from build123d import *

# Parameters (mm, degrees)
SKETCH1_W               = 5
SKETCH1_H               = 13
SKETCH1_R               = 1.25
BOSS_EXTRUDE1_DEPTH     = 2.5
BOSS_EXTRUDE1_2_DEPTH   = 2.5
SKETCH1_5_W             = 32.5
SKETCH1_5_H             = 2
BOSS_EXTRUDE2_DEPTH     = 20.5
SKETCH1_6_W             = 32.5
SKETCH1_6_H             = 3
BOSS_EXTRUDE3_DEPTH     = 3.5
SKETCH2_R               = 1.5
CUT_EXTRUDE2_DEPTH      = 14
CUT_EXTRUDE2_DEPTH_BACK = 8


with BuildPart() as part:
    # Sketch1 → Boss-Extrude1 (new body)
    with BuildSketch(Plane.XY):
        with Locations((-13.75, 6.5)):
            Rectangle(SKETCH1_W, SKETCH1_H)
        with Locations((-13.75, 6)):
            Circle(SKETCH1_R, mode=Mode.SUBTRACT)
    extrude(amount=BOSS_EXTRUDE1_DEPTH)



with BuildPart() as body_2:
    # Sketch1 → Boss-Extrude1 2 (new body)
    with BuildSketch(Plane.XY):
        with Locations((13.75, 6.5)):
            Rectangle(SKETCH1_W, SKETCH1_H)
        with Locations((13.75, 6)):
            Circle(SKETCH1_R, mode=Mode.SUBTRACT)
    extrude(amount=BOSS_EXTRUDE1_2_DEPTH)


with BuildPart() as part_1:
    add(part.part)

    add(body_2.part)  # Boss-Extrude2 merges body 2
    # Sketch1<5> → Boss-Extrude2 (add)
    with BuildSketch(Plane.XY):
        with Locations((0, -1)):
            Rectangle(SKETCH1_5_W, SKETCH1_5_H)
        with Locations((0, -6)):
            Rectangle(SKETCH1_5_W, SKETCH1_5_H)
    extrude(amount=BOSS_EXTRUDE2_DEPTH)

    # Sketch1<6> → Boss-Extrude3 (add)
    with BuildSketch(Plane.XY):
        with Locations((0, -3.5)):
            Rectangle(SKETCH1_6_W, SKETCH1_6_H)
    extrude(amount=BOSS_EXTRUDE3_DEPTH)

    # Sketch2 → Cut-Extrude2 (cut, two sides)
    with BuildSketch(Plane(origin=(0, 0, 0), x_dir=(1, 0, 0), z_dir=(0, 1, 0))) as cut_extrude2_sk:
        with Locations((13.75, -8.5)):
            Circle(SKETCH2_R)
        with Locations((13.75, -15.5)):
            Circle(SKETCH2_R)
        with Locations((-13.75, -15.5)):
            Circle(SKETCH2_R)
        with Locations((-13.75, -8.5)):
            Circle(SKETCH2_R)
    extrude(amount=CUT_EXTRUDE2_DEPTH, mode=Mode.SUBTRACT)
    extrude(cut_extrude2_sk.sketch, amount=-CUT_EXTRUDE2_DEPTH_BACK, mode=Mode.SUBTRACT)


solid = part_1.part
Geometry: final body of the model. Coordinates: model frame, mm. A direction names the side the tool comes from. Coordinates: 2 decimals unless noted, no trailing zeros. Write each loop counter-clockwise with the first axis right and the second up, starting at its lowest first coordinate (ties: lowest second). Pieces come first, ordered by that corner, then holes. Notation, with made-up numbers: (2.5, 5) - (53.5, 5) arc R19 ccw to (53.5, 22) - close; hole circle Ø10 at (-13.5, 74.5). An arc over 180 degrees is marked (long way). Return JSON: item names as keys, results as strings.
Item 1: Line query: L1, parallel to X at y = -0.95, z = 8.5; L2, parallel to Z at x = -13.75, y = -1.2; L3, parallel to Y at x = 10, z = 17.25. Output: solid intervals per line, ascending.
Completed:
{"L1": "x = -16.25 to -15.25, -12.25 to 12.25, 15.25 to 16.25", "L2": "z = 0 to 7, 10 to 14, 17 to 20.5", "L3": "y = -7 to -5, -2 to 0"}
Item 2: Section query A-A (z = 19). Output: boundary loops of the cut face in (x, y), and give its area (3 significant figures).
Completed:
{"outline": "(-16.25, -7) - (16.25, -7) - (16.25, -5) - (-16.25, -5) - close; (-16.25, -2) - (16.25, -2) - (16.25, 0) - (-16.25, 0) - close", "area": "130 mm2"}
Item 3: Section query B-B (y = 2.75). Output: boundary loops of the cut face in (x, z), and give its area (3 significant figures).
Completed:
{"outline": "(-16.25, 0) - (-11.25, 0) - (-11.25, 2.5) - (-16.25, 2.5) - close; (11.25, 0) - (16.25, 0) - (16.25, 2.5) - (11.25, 2.5) - close", "area": "25.0 mm2"}
Item 4: Pull-direction query (X, two-part tool) for faces 1 (the face through (-14, 13, 1)), 2 (the face through (16.25, -1, 8)), 3 (the face through (12.56, -0.99, 9.41)); classes: +X half, -X half, draft (parallel to the pull), parting line (faces both ways), or undercut.
Completed:
{"face 1": "draft", "face 2": "+X half", "face 3": "undercut"}
Item 5: Section query D-D (z = 15.5). Output: boundary loops of the cut face in (x, y).
Completed:
{"outline": "(-16.25, -7) - (-15.25, -7) - (-15.25, -5) - (-16.25, -5) - close; (-16.25, -2) - (-15.25, -2) - (-15.25, 0) - (-16.25, 0) - close; (-12.25, -7) - (12.25, -7) - (12.25, -5) - (-12.25, -5) - close; (-12.25, -2) - (12.25, -2) - (12.25, 0) - (-12.25, 0) - close; (15.25, -7) - (16.25, -7) - (16.25, -5) - (15.25, -5) - close; (15.25, -2) - (16.25, -2) - (16.25, 0) - (15.25, 0) - close"}
Item 6: Section query C-C (x = -13.75). Count the separate pieces of the cut face and the enclosed holes in it, and give its area (4 significant figures).
Completed:
{"separate pieces": "6", "enclosed holes": "0", "area": "94.75 mm2"}
Item 7: Reachability of faces 4 (the face through (11.25, 6, 1)), 5 (the face through (0, -3, 3.5)), 6 (the face through (12.25, -5.99, 15.43)), 7 (the face through (14, 8, 2.5)), 8 (the face through (0, -1, 20.5)) from +Z, -Z, +X, -X, +Y, -Y: full face, straight path, thin tool, end or side. Return the list, or none.
Completed:
{"face 4": "+Z, -Z, +Y", "face 5": "+Z, +X, -X", "face 6": "+Y, -Y", "face 7": "+Z, +X, -X, +Y", "face 8": "+Z, +X, -X, +Y, -Y"}
Item 8: Pin query (flat end, axial travel): pin 1 Ø4 at (x, z) = (-13.75, 8.5) entering from -Y; pin 2 Ø1.5 at (y, z) = (3.5, 5) entering from +X; pin 3 Ø3 at (x, z) = (7, 3.5) entering from +Y; pin 4 Ø1.5 at (x, y) = (-4.5, -3.5) entering from +Z. Return the tip coordinate at first contact, or that it passes through.
Completed:
{"pin 1": "stops at y = -7", "pin 2": "passes through", "pin 3": "stops at y = 0", "pin 4": "stops at z = 3.5"}
